Input: part model. Units: mm. Frame: model coordinates. A direction names the side the tool comes from. Give positions to 0.01 mm unless a question says otherwise; leave off trailing zeros. Order: outer loops, then holes, each group sorted by start corner. A loop starts at its lowest first (then second) coordinate and runs counter-clockwise, first axis right, second up. Notation, with made-up numbers: (-12, 61.5) - (-8, 61.5) arc R22 cw to (-8, 67.5) - close; hole circle Ø6 at (-29.75, 59). An arc over 180 degrees is marked (long way). Use a Markdown table: item, result.
from build123d import *

# Parameters (mm, degrees)
SKETCH1_R           = 3.875
BOSS_EXTRUDE1_DEPTH = 20
SKETCH2_OUTSIDE_W   = 14.312
SKETCH2_OUTSIDE_H   = 14.312
SKETCH2_OUTSIDE_R   = 2.39
CUT_EXTRUDE1_DEPTH  = 15
CHAMFER1_SIZE       = 0.5
CUT_EXTRUDE2_DEPTH  = 3.36


with BuildPart() as part:
    # Sketch1 → Boss-Extrude1 (new body)
    with BuildSketch(Plane(origin=(0, 0, 0), x_dir=(1, 0, 0), z_dir=(0, 1, 0))):
        with Locations(Location((0, 0, 0), (0, 0, 270))):
            Circle(SKETCH1_R)
    extrude(amount=BOSS_EXTRUDE1_DEPTH)

    # Sketch2 outside → Cut-Extrude1 (cut)
    with BuildSketch(Plane(origin=(0, 20, 0), x_dir=(1, 0, 0), z_dir=(0, 1, 0))):
        Rectangle(SKETCH2_OUTSIDE_W, SKETCH2_OUTSIDE_H)
        with Locations(Location((0, 0, 0), (0, 0, 270))):
            Circle(SKETCH2_OUTSIDE_R, mode=Mode.SUBTRACT)
    extrude(amount=-CUT_EXTRUDE1_DEPTH, mode=Mode.SUBTRACT)

    # Chamfer1
    chamfer1_edges = [part.edges().sort_by_distance(p)[0] for p in [
        (0, 20, -2.39),
    ]]
    chamfer(chamfer1_edges, length=CHAMFER1_SIZE)

    # Sketch8 → Cut-Extrude2 (cut)
    with BuildSketch(Plane.XZ):
        Polygon((2.644264233, 0), (1.322132116, 2.29), (-1.322132116, 2.29), (-2.644264233, 0), (-1.322132116, -2.29), (1.322132116, -2.29), align=None)
    extrude(amount=-CUT_EXTRUDE2_DEPTH, mode=Mode.SUBTRACT)


solid = part.part
1. Section query A-A (y = 2). Return loops of the section in (x, z) (3 decimals).
Response:
| item | result |
|---|---|
| outline | circle Ø7.75 at (0, 0); hole (-2.644, 0) - (-1.322, -2.29) - (1.322, -2.29) - (2.644, 0) - (1.322, 2.29) - (-1.322, 2.29) - close |
2. Section query D-D (x = 3). Return loops of the section in (y, z).
Response:
| item | result |
|---|---|
| outline | (0, -2.45) - (5, -2.45) - (5, 2.45) - (0, 2.45) - close |
3. Pin query (flat end, axial travel): pin 1 (2 mm diameter, centred on x = -0.5, y = 1, fed in from +Z) (3 decimals); pin 2 (3 mm diameter, centred on x = 0, y = 17.5, fed in from +Z); pin 3 (2 mm diameter, centred on y = 9, z = 3, fed in from -X); pin 4 (1.5 mm diameter, centred on y = 15.5, z = 0.5, fed in from +X). Return the tip coordinate at first contact, or that it passes through.
Response:
| item | result |
|---|---|
| pin 1 | stops at z = 3.875 |
| pin 2 | stops at z = 2.39 |
| pin 3 | stops at x = -1.31 |
| pin 4 | stops at x = 2.39 |
4. Material intervals for line 1 along Y through (x, z) = (2.75, -2.25); line 2 along Y through (x, z) = (-0.5, 0.5); line 3 along Z through (x, y) = (0, 3.25) (3 decimals), sorted ascending.
Response:
| item | result |
|---|---|
| line 1 | y = 0 to 5 |
| line 2 | y = 3.36 to 20 |
| line 3 | z = -3.875 to -2.29, 2.29 to 3.875 |
5. Section query B-B (x = 0). Return loops of the section in (y, z) (3 decimals).
Response:
| item | result |
|---|---|
| outline | (0, -3.875) - (5, -3.875) - (5, -2.39) - (19.5, -2.39) - (20, -1.89) - (20, 1.89) - (19.5, 2.39) - (5, 2.39) - (5, 3.875) - (0, 3.875) - (0, 2.29) - (3.36, 2.29) - (3.36, -2.29) - (0, -2.29) - close |
6. Set-up query: faces 1 (the face through (3.842, 2.465, -0.504)), 2 (the face through (-1.99, 1.66, -1.13)), 3 (the face through (1.615, 12.352, -1.762)). Return all of +Z, -Z, +X, -X, +Y, -Y with unobstructed straight access to the full face (end or side cutting, diameter ignored); none if empty.
Response:
| item | result |
|---|---|
| face 1 | +Y, -Y |
| face 2 | -Y |
| face 3 | +Y |
7. Section query C-C (y = 14). Return loops of the section in (x, z), then the cut area to 3 significant figures.
Response:
| item | result |
|---|---|
| outline | circle Ø4.78 at (0, 0) |
| area | 17.9 mm^2 |
